For this review, take the finished solid that the model builds, in its own axes (mm). Round coordinates to 2 decimals unless told otherwise and drop trailing zeros. Answer in a Markdown table with one row per item.
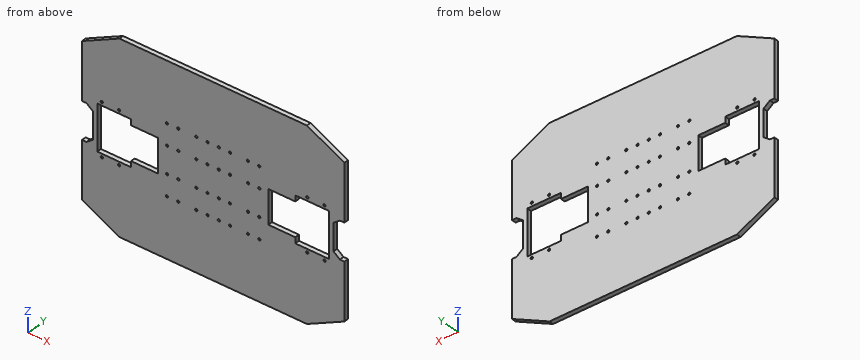
Autodesk Inventor part; units mm, degrees
ref_plane "YZ Plane" through (0, 0, 0) normal (1, 0, 0) x (0, 1, 0)
ref_plane "XZ Plane" through (0, 0, 0) normal (0, 1, 0) x (-1, 0, 0)
ref_plane "XY Plane" through (0, 0, 0) normal (0, 0, 1) x (1, 0, 0)
sketch "BodySketch" plane through (0, 0, 0) normal (0, 1, 0) x (-1, 0, 0)
  line L0 (0, 125) -> (125, 125)
  line L1 (125, 125) -> (175, 100)
  line L2 (175, 100) -> (175, 24.5)
  line L3 (175, 24.5) -> (169, 24.5)
  line L4 (160.5, 18) -> (160.5, -18)
  line L5 (169, -24.5) -> (175, -24.5)
  line L6 (175, -24.5) -> (175, -100)
  line L7 (175, -100) -> (125, -125)
  line L8 (125, -125) -> (0, -125)
  line L9 (0, 0) -> (0, 145.614) construction
  line L10 (0, 125) -> (-125, 125)
  line L11 (-125, 125) -> (-175, 100)
  line L12 (-175, 100) -> (-175, 24.5)
  line L13 (-175, -24.5) -> (-175, -100)
  line L14 (-175, -100) -> (-125, -125)
  line L15 (-125, -125) -> (0, -125)
  line L16 (0, 0) -> (316.974, 0) construction
  line L17 (160.5, 18) -> (169, 24.5)
  line L18 (160.5, -18) -> (169, -24.5)
  line L19 (-175, 24.5) -> (-169, 24.5)
  line L20 (-160.5, 18) -> (-160.5, -18)
  line L21 (-169, -24.5) -> (-175, -24.5)
  line L22 (-160.5, 18) -> (-169, 24.5)
  line L23 (-160.5, -18) -> (-169, -24.5)
  point P0 (160.5, 24.5)
  point P1 (160.5, -24.5)
  dimension "Chassis_Body_Width" = 350
  dimension "Chassis_Body_Length" = 250
  dimension "Chassis_EncoderWheelSpace_Diameter" = 49
  dimension "Chassis_EncoderWheelSpace_Width" = 14.5
  dimension "Chassis_Body_InnerLength" = 200
  dimension "Chassis_Body_InnerWidth" = 250
  dimension "d14" = 6
  dimension "d15" = 36
extrude "Body" add sketch "BodySketch" along normal blind 6
sketch "EncoderBodyHoleSketch" plane through (0, 6, 0) normal (0, 1, 0) x (1, 0, 0)
  line L0 (-175, 100) -> (-175, 24.5)
  line L1 (-175, -24.5) -> (-175, -100)
  line L2 (0, 0) -> (0, 145.3586) construction
  line L3 (-154.5, 30.25) -> (-109.5, 30.25)
  line L4 (-109.5, 30.25) -> (-109.5, -30.25)
  line L5 (-109.5, -30.25) -> (-154.5, -30.25)
  line L6 (-154.5, -30.25) -> (-154.5, 30.25)
  line L7 (0, 0) -> (187.4589, 0) construction
  line L8 (154.5, 30.25) -> (109.5, 30.25)
  line L9 (109.5, 30.25) -> (109.5, -30.25)
  line L10 (109.5, -30.25) -> (154.5, -30.25)
  line L11 (154.5, -30.25) -> (154.5, 30.25)
  line L12 (-169, -24.5) -> (-175, -24.5)
  line L13 (-132, 0) -> (-132, 72.6793) construction
  point P0 (-160.5, -24.5)
  dimension "d9" = 45
  dimension "d10" = 60.5
  dimension "d13" = 43
extrude "EncoderBodyHole" cut sketch "EncoderBodyHoleSketch" against normal up to next
sketch "EncoderSupportFasteningSketch" plane through (0, 6, 0) normal (0, 1, 0) x (1, 0, 0)
  line L0 (-175, 100) -> (-175, 24.5)
  line L1 (-175, -24.5) -> (-175, -100)
  line L2 (0, 0) -> (0, 103.2036) construction
  line L3 (-120.5, 39.75) -> (-153.5, 39.75) construction
  line L4 (-153.5, 39.75) -> (-153.5, -39.75) construction
  line L5 (-153.5, -39.75) -> (-120.5, -39.75) construction
  line L6 (-120.5, -39.75) -> (-120.5, 39.75) construction
  line L7 (0, 0) -> (196.594, 0) construction
  circle A0 centre (-148.5, 34.75) radius 1.5
  circle A1 centre (-148.5, -34.75) radius 1.5
  line L8 (-137, 47.3947) -> (-137, -51.0004) construction
  circle A2 centre (-125.5, 34.75) radius 1.5
  circle A3 centre (-125.5, -34.75) radius 1.5
  circle A4 centre (148.5, 34.75) radius 1.5
  circle A5 centre (148.5, -34.75) radius 1.5
  circle A6 centre (125.5, 34.75) radius 1.5
  circle A7 centre (125.5, -34.75) radius 1.5
  dimension "d16" = 79.5
  dimension "d17" = 33
  dimension "d18" = 21.5
  dimension "d19" = 3
  dimension "d20" = 5
  dimension "d21" = 5
  dimension "d22" = 16.5
extrude "EncoderSupportFastening" cut sketch "EncoderSupportFasteningSketch" against normal up to next
sketch "MotorBlockFasteningSketch" plane through (0, 6, 0) normal (0, 1, 0) x (1, 0, 0)
  line L0 (10.676, -18) -> (24.3135, -18) construction
  circle A0 centre (7.5, -18) radius 1.5
  circle A1 centre (22.5, -18) radius 1.5
  line L1 (0, 0) -> (0, -28.6489) construction
  circle A2 centre (46.5, -18) radius 1.5
  circle A3 centre (61.5, -18) radius 1.5
  circle A4 centre (7.5, -46) radius 1.5
  circle A5 centre (22.5, -46) radius 1.5
  circle A6 centre (46.5, -46) radius 1.5
  circle A7 centre (61.5, -46) radius 1.5
  circle A8 centre (-7.5, -18) radius 1.5
  circle A9 centre (-22.5, -18) radius 1.5
  circle A10 centre (-46.5, -18) radius 1.5
  circle A11 centre (-61.5, -18) radius 1.5
  circle A12 centre (-7.5, -46) radius 1.5
  circle A13 centre (-22.5, -46) radius 1.5
  circle A14 centre (-46.5, -46) radius 1.5
  circle A15 centre (-61.5, -46) radius 1.5
  line L2 (0, 0) -> (72.0385, 0) construction
  circle A16 centre (7.5, 18) radius 1.5
  circle A17 centre (22.5, 18) radius 1.5
  line L3 (0, 0) -> (0, 28.6489) construction
  circle A18 centre (46.5, 18) radius 1.5
  circle A19 centre (61.5, 18) radius 1.5
  circle A20 centre (7.5, 46) radius 1.5
  circle A21 centre (22.5, 46) radius 1.5
  circle A22 centre (46.5, 46) radius 1.5
  circle A23 centre (61.5, 46) radius 1.5
  circle A24 centre (-7.5, 18) radius 1.5
  circle A25 centre (-22.5, 18) radius 1.5
  circle A26 centre (-46.5, 18) radius 1.5
  circle A27 centre (-46.5, 46) radius 1.5
  circle A28 centre (-61.5, 18) radius 1.5
  circle A29 centre (-61.5, 46) radius 1.5
  circle A30 centre (-7.5, 46) radius 1.5
  circle A31 centre (-22.5, 46) radius 1.5
  dimension "d25" = 3
  dimension "d28" = 15
  dimension "d35" = 39
  dimension "d38" = 28
  dimension "d41" = 15
  dimension "d46" = 18
extrude "MotorBlockFastening" cut sketch "MotorBlockFasteningSketch" against normal up to next
sketch "MotorWheelHoleSketch" plane through (0, 6, 0) normal (0, 1, 0) x (1, 0, 0)
  line L0 (-109.5, 30.25) -> (-109.5, -30.25)
  line L1 (-109.5, 22.5) -> (-73.5, 22.5)
  line L2 (-73.5, 22.5) -> (-73.5, -22.5)
  line L3 (-73.5, -22.5) -> (-109.5, -22.5)
  line L4 (-109.5, -22.5) -> (-109.5, 22.5)
  line L5 (0, 0) -> (72.3504, 0) construction
  line L6 (-175, -24.5) -> (-175, -100)
  line L7 (0, 0) -> (0, 70.7306) construction
  line L8 (109.5, 22.5) -> (73.5, 22.5)
  line L9 (73.5, 22.5) -> (73.5, -22.5)
  line L10 (73.5, -22.5) -> (109.5, -22.5)
  line L11 (109.5, -22.5) -> (109.5, 22.5)
  dimension "d49" = 36
  dimension "d50" = 45
extrude "MotorWheelHole" cut sketch "MotorWheelHoleSketch" against normal up to next
equation "\"Chassis_EncoderWheelSpace_Diameter\" = EncoderWheel_Tyre_Diameter"
equation "\"Chassis_EncoderWheelSpace_Width\" = EncoderBlock_InterfaceToWheel_Distance + Chassis_MecanicalSpace"
equation "\"d14\" = EncoderWheel_Tyre_Width"
equation "\"d15\" = EncoderWheelInterface_Diameter"
equation "\"d9\" = EncoderSupportInside_Front_Thickness + Encoder_Body_Length + 2 * Chassis_MecanicalSpace"
equation "\"d10\" = EncoderSupportInside_Width + 2 * Chassis_MecanicalSpace"
equation "\"d13\" = EncoderBlock_SupportToWheel_Distance + 0.5 * Encoder_Body_Length + 0.5 * EncoderSupportInside_Front_Thickness"
equation "\"d16\" = EncoderSupportOutside_Width"
equation "\"d17\" = EncoderSupportOutside_Length"
equation "\"d18\" = EncoderBlock_SupportToWheel_Distance"
equation "\"d19\" = EncoderSupport_FixingHole_Diameter"
equation "\"d20\" = EncoderSupport_FixingnHole_Margin"
equation "\"d21\" = EncoderSupport_FixingnHole_Margin"
equation "\"d22\" = 0.5 * EncoderSupportOutside_Length"
equation "\"d28\" = Bracket_Holes_Distance"
equation "\"d35\" = Bracket_Holes_Distance + Bracket_Holes_UnfoldedDistance"
equation "\"d38\" = Bracket_Holes_LateralDistance"
equation "\"d41\" = Bracket_Holes_Distance"
equation "\"d46\" = Motor_FasteningHole_DistanceToCenter"
equation "\"Chassis_MecanicalSpace\" = 1"
properties part number "Chassis" material "Wood (Oak)"
1) Clearance check with flat-ended pins moving along their axes: pin 1 Ø3 at (x, y) = (170.5, 4) entering from +Z; pin 2 Ø5 at (x, z) = (148.5, -34.75) entering from +Y; pin 3 Ø1.8 at (x, z) = (-148.5, 34.75) entering from +Y; pin 4 Ø3 at (x, y) = (-139.5, 3.5) entering from +Z. State where each tip first meets the part, or that it passes through.
Solved:
| item | result |
|---|---|
| pin 1 | z = 103 |
| pin 2 | y = 6 |
| pin 3 | through |
| pin 4 | z = 118.5 |
2) Consider section A-A on y = 1.9. State how many separate pieces and enclosed holes the cut face has, then the cut area to 3 significant figures.
Solved:
| item | result |
|---|---|
| separate pieces | 1 |
| enclosed holes | 42 |
| area | 74,700 mm² |
3) For line 1 (X direction, y = 3.65, z = 27); line 2 (Z direction, x = -22.5, y = 2.95); line 3 (Z direction, x = 114, y = 4.7), list the stretches that pass through material, from the lowest coordinate up. Write a range as [from, to].
Solved:
| item | result |
|---|---|
| line 1 | [-175, -154.5], [-109.5, 109.5], [154.5, 175] |
| line 2 | [-125, -47.5], [-44.5, -19.5], [-16.5, 16.5], [19.5, 44.5], [47.5, 125] |
| line 3 | [-125, -30.25], [30.25, 125] |
